```python
from build123d import *


with BuildPart() as part:
    # Sketch1 → Revolve1 (revolve)
    with BuildSketch(Plane.XY):
        with BuildLine():
            Line((0, 5.35), (0, 4.767))
            Line((0, 4.767), (0.12, 4.767))
            Line((0.12, 4.767), (0.12, 3.46))
            Line((0.12, 3.46), (0, 3.46))
            Line((0, 3.46), (0, 2.65))
            ThreePointArc((0, 2.65), (0.043933983, 2.543933983), (0.15, 2.5))
            Line((0.15, 2.5), (4.85, 2.5))
            ThreePointArc((4.85, 2.5), (4.956066017, 2.543933983), (5, 2.65))
            Line((5, 2.65), (5, 3.46))
            Line((5, 3.46), (4.88, 3.46))
            Line((4.88, 3.46), (4.88, 4.767))
            Line((4.88, 4.767), (5, 4.767))
            Line((5, 4.767), (5, 5.35))
            ThreePointArc((5, 5.35), (4.956066017, 5.456066017), (4.85, 5.5))
            Line((4.85, 5.5), (0.15, 5.5))
            ThreePointArc((0.15, 5.5), (0.043933983, 5.456066017), (0, 5.35))
        make_face()
    revolve(axis=Axis((4.85, 0, 0), (-1, 0, 0)))


solid = part.part
```
Design review of the part built by this model. Coordinates are the model's own, in mm. Coordinates: 2 decimals unless noted, no trailing zeros. Order: outer loops, then holes, each group sorted by start corner. A loop starts at its lowest first (then second) coordinate and runs counter-clockwise, first axis right, second up.
1) Clearance check with flat-ended pins moving along their axes: pin 1 (1 mm diameter, centred on x = 2, z = 1.5, fed in from +Y); pin 2 (2 mm diameter, centred on x = 3.5, y = -4, fed in from -Z). State where each tip first meets the part, or that it passes through.
2) Take a section at C-C, the plane x = 3.15. Give the boundary of the cut face in (y, z).
3) Mouldability with a two-part tool opening along Z and no side actions: class faces 1 (the flat face through (0.12, 0, -4)), 2 (the cylindrical face through (2.47, -1.19, 5.37)), 3 (the flat face through (4.88, 0, -4)), 4 (the flat face through (5, 4, 3)) as +Z half, -Z half, draft (parallel to the pull), parting line (faces both ways), or undercut.
4) Wall thickness on line 1 along Z through (x, y) = (2.3, 0); line 2 along Y through (x, z) = (0.05, 0): over which ranges is each line inside the solid? List them lowest first.
Returned:
1. pin 1: stops at y = 5.41
1. pin 2: stops at z = -4.61
2. outline: circle Ø11 at (0, 0); hole circle Ø5 at (0, 0)
3. face 1: undercut
3. face 2: parting line
3. face 3: undercut
3. face 4: draft
4. line 1: z = -5.5 to -2.5, 2.5 to 5.5
4. line 2: y = -5.46 to -4.77, -3.46 to -2.54, 2.54 to 3.46, 4.77 to 5.46
